from build123d import *

# Parameters (mm, degrees)
SKETCH1_R           = 4
BOSS_EXTRUDE1_DEPTH = 65
SKETCH2_R           = 1.3
CUT_EXTRUDE1_DEPTH  = 66.245689513


with BuildPart() as part:
    # Sketch1 → Boss-Extrude1 (new, symmetric)
    with BuildSketch(Plane.XY):
        Circle(SKETCH1_R)
    extrude(amount=BOSS_EXTRUDE1_DEPTH, both=True)

    # Sketch2 → Cut-Extrude1 (cut, symmetric)
    with BuildSketch(Plane(origin=(0, 0, 0), x_dir=(0, 0, -1), z_dir=(1, 0, 0))):
        with Locations((56.5, 0)):
            Circle(SKETCH2_R)
    cut_extrude1 = extrude(amount=CUT_EXTRUDE1_DEPTH, both=True, mode=Mode.SUBTRACT)

    # Mirror1: Cut-Extrude1 across plane
    add(cut_extrude1.mirror(Plane.XY), mode=Mode.SUBTRACT)


solid = part.part
Input: part model. Units: mm. Frame: model coordinates. Give positions to 0.01 mm unless a question says otherwise; leave off trailing zeros. Order: outer loops, then holes, each group sorted by start corner. A loop starts at its lowest first (then second) coordinate and runs counter-clockwise, first axis right, second up. Notation, with made-up numbers: (-20, -25) - (-3, -25) arc R25 ccw to (-3, -9) - close; hole circle Ø4 at (69.25, 0.25). An arc over 180 degrees is marked (long way). Answer as a JSON object with one key per item and string values. Group by question number.
Q1. Cut plane C-C, the plane z = 41.5. Output: boundary loops of the cut face in (x, y), then the cut area to 3 significant figures.
Q2. Mould query, pull axis Y, two halves, no side actions, for faces 1 (the face through (-0.867, -3.905, 0.91)), 2 (the face through (0.06, 0.39, -57.74)), 3 (the face through (0, 0, -65)). Classes: pulls with the +Y half, pulls with the -Y half, needs draft (parallel to the pull), parting line crosses it, or undercut.
Q3. Cut plane A-A, the plane y = 0. Output: boundary loops of the cut face in (x, z).
Q4. First-contact query: pin 1 Ø1 at (x, z) = (-1.5, 8) entering from -Y; pin 2 Ø1 at (x, z) = (-2.5, 24.5) entering from +Y. Flat tips, straight axial feed; report the tip coordinate or a pass-through.
Q5. Cut plane B-B, the plane x = 1. Output: boundary loops of the cut face in (y, z).
Q6. Line query: probe 1 along Z at (x, y) = (0.25, 0); probe 2 along Z at (x, y) = (3.5, -0.75); probe 3 along Y at (x, z) = (-0.5, 56.5). Output: solid intervals per line, ascending.
Q7. Cut plane D-D, the plane z = -56.5. Output: boundary loops of the cut face in (x, y).
Results:
{
 "1": {"outline": "circle Ø8 at (0, 0)", "area": "50.3 mm^2"},
 "2": {"face 1": "parting line crosses it", "face 2": "undercut", "face 3": "needs draft"},
 "3": {"outline": "(-4, -65) - (4, -65) - (4, -57.8) - (-4, -57.8) - close; (-4, -55.2) - (4, -55.2) - (4, 55.2) - (-4, 55.2) - close; (-4, 57.8) - (4, 57.8) - (4, 65) - (-4, 65) - close"},
 "4": {"pin 1": "y = -3.87", "pin 2": "y = 3.46"},
 "5": {"outline": "(-3.87, -65) - (3.87, -65) - (3.87, 65) - (-3.87, 65) - close; hole circle Ø2.6 at (0, -56.5); hole circle Ø2.6 at (0, 56.5)"},
 "6": {"probe 1": "-65 to -57.8, -55.2 to 55.2, 57.8 to 65", "probe 2": "-65 to -57.56, -55.44 to 55.44, 57.56 to 65", "probe 3": "-3.97 to -1.3, 1.3 to 3.97"},
 "7": {"outline": "(-3.78, -1.3) arc R4 ccw to (3.78, -1.3) - close; (-3.78, 1.3) - (3.78, 1.3) arc R4 ccw to start"}
}
